For this review, use the dimensioned drawing (mm, ordinates from the lowest corner) and the shaded views. Give positions to 0.01 mm unless a question says otherwise; leave off trailing zeros. Order: outer loops, then holes, each group sorted by start corner. A loop starts at its lowest first (then second) coordinate and runs counter-clockwise, first axis right, second up.
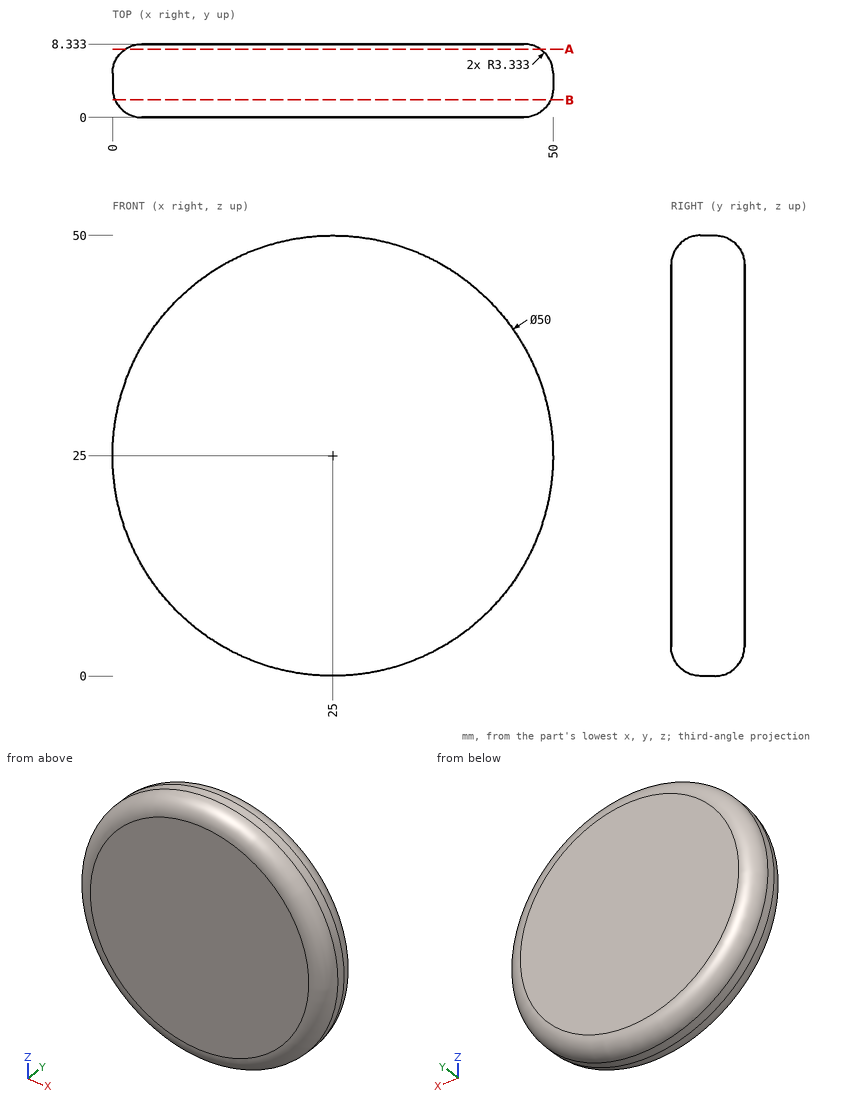
1. For pin 1 (3 mm diameter, centred on x = 12, y = 4.5, fed in from +Z); pin 2 (1.5 mm diameter, centred on y = 6.5, z = 25, fed in from +X) (1 decimal); pin 3 (2 mm diameter, centred on x = 20.5, y = 5.5, fed in from -Z), all flat-tipped, find the tip position at first contact; note any pin that passes through.
Recorded:
pin 1: stops at z = 47.2
pin 2: stops at x = 49.9
pin 3: stops at z = 0.26
2. Take a section at B-B (y = 2). State the section outline as (x, z) points, then the cut area to 3 significant figures.
Recorded:
outline: circle Ø49.44 at (25, 25)
area: 1,920 mm2
3. Take a section at A-A (y = 7.75). State the section outline as (x, z) points, then the cut area to 3 significant figures.
Recorded:
outline: circle Ø47.1 at (25, 25)
area: 1,740 mm2
4. For line 1 along X through (y, z) = (4, 25); line 2 along Y through (x, z) = (4, 16) (1 decimal); line 3 along X through (y, z) = (7.75, 21), list the stretches that pass through material, from the lowest coordinate up.
Recorded:
line 1: x = 0 to 50
line 2: y = 0.2 to 8.1
line 3: x = 1.79 to 48.21
